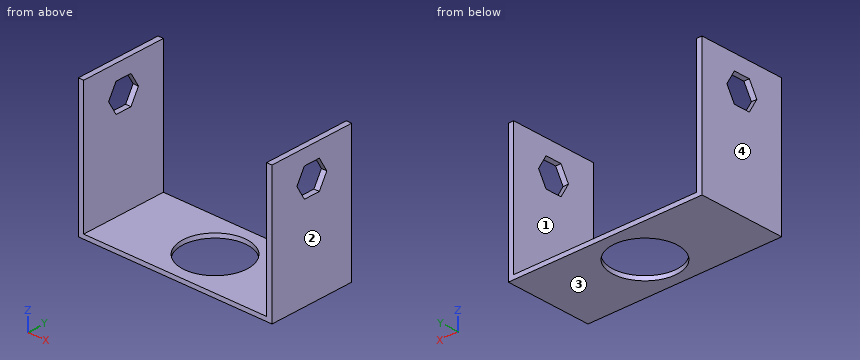
Autodesk Inventor part; units mm, degrees
ref_plane "Work Plane2" through (110.8745, -46.6041, 76.2) normal (1, 0, 0) x (0, 0, -1)
ref_plane "YZ Plane" through (0, 0, 0) normal (1, 0, 0) x (0, 1, 0)
ref_plane "XZ Plane" through (0, 0, 0) normal (0, 1, 0) x (-1, 0, 0)
sketch "Sketch1" plane through (0, 0, 0) normal (0, 0, 1) x (1, 0, 0)
  line L0 (-3.4255, 4.1959) -> (110.8745, 4.1959)
  line L1 (110.8745, 4.1959) -> (110.8745, -46.6041)
  line L2 (110.8745, -46.6041) -> (-3.4255, -46.6041)
  line L3 (-3.4255, -46.6041) -> (-3.4255, 4.1959)
  circle A0 centre (53.7245, -21.2041) radius 19.05
  line L4 (-0.2505, 4.1959) -> (-0.2505, -46.6041)
  line L5 (107.6995, -46.6041) -> (107.6995, 4.1959)
  point P0 (0, 0)
  dimension "d0" = 114.3
  dimension "d1" = 50.8
  dimension "d2" = 38.1
  dimension "d3" = 57.15
  dimension "d4" = 25.4
  dimension "d5" = 3.175
  dimension "d6" = 3.175
extrude "Extrusion1" add sketch "Sketch1" along normal blind 76.2 contours L0 L4 L2 L3 | L0 L1 L2 L5
extrude "Extrusion2" add sketch "Sketch1" against normal blind 2.54
ref_plane "Work Plane2" through (110.8745, -46.6041, 76.2) normal (1, 0, 0) x (0, 0, -1)
sketch "Sketch3" plane through (110.8745, -46.6041, 76.2) normal (1, 0, 0) x (0, 0, -1)
  line L0 (8.888, 20.6375) -> (8.888, 30.1625)
  line L1 (8.888, 30.1625) -> (17.1369, 34.925)
  line L2 (17.1369, 34.925) -> (25.3858, 30.1625)
  line L3 (25.3858, 30.1625) -> (25.3858, 20.6375)
  line L4 (25.3858, 20.6375) -> (17.1369, 15.875)
  line L5 (17.1369, 15.875) -> (8.888, 20.6375)
  line L6 (0, 0) -> (0, 50.8)
  line L7 (78.74, 0) -> (0, 0)
  point P0 (76.2, 46.6041)
  dimension "d12" = 9.525
  dimension "d13" = 9.525
  dimension "d14" = 120
  dimension "d15" = 9.525
  dimension "d16" = 120
  dimension "d17" = 9.525
  dimension "d18" = 120
  dimension "d19" = 8.888
  dimension "d20" = 15.875
extrude "Extrusion3" cut sketch "Sketch3" against normal blind 127
properties part number "shaft to bicep" material "CFRP"
Design review of the part built by this model. Coordinates are the model's own, in mm. Face numbers are marked on the shaded views. Round coordinates to 2 decimals unless told otherwise and drop trailing zeros. Loops run counter-clockwise (first coordinate to the right, second up) from the corner with the lowest first, then second, coordinate; pieces in that order, holes last. Notation, with made-up numbers: (59, 75) -> (82, 75) arc R15 cw to (82, 89) -> close; hole circle Ø1 at (59.25, -23). An arc over 180 degrees is marked (long way). Use one line per item in the form item = value. Start each with the question number.
Q1. We need section D-D on y = -9.5. Give the boundary of the cut face in (x, z).
Q2. We need section C-C on y = -15. Give the boundary of the cut face in (x, z), then the cut area to 3 significant figures.
Q3. Draft analysis for pull direction X (two halves, no side actions). For the marked faces 1, 2, 3 and 4, state which applies: +X half, -X half, draft (parallel to the pull), parting line (faces both ways), or undercut.
Q4. We need section B-B on x = 49.5. Give the boundary of the cut face in (y, z), then the cut area to 3 significant figures.
Q5. Wall thickness on line 1 along X through (y, z) = (-39, 3.5); line 2 along Z through (x, y) = (88, -10.5): over which ranges is each line inside the solid? List them lowest first. Write a range as [from, to].
Q6. We need section A-A on z = 4.5. Give the boundary of the cut face in (x, y), then the cut area to 3 significant figures.
Calculated:
q1.outline = (-3.43, -2.54) -> (38.69, -2.54) -> (38.69, 0) -> (-0.25, 0) -> (-0.25, 76.2) -> (-3.43, 76.2) -> close; (68.76, -2.54) -> (110.87, -2.54) -> (110.87, 76.2) -> (107.7, 76.2) -> (107.7, 0) -> (68.76, 0) -> close
q2.outline = (-3.43, -2.54) -> (35.71, -2.54) -> (35.71, 0) -> (-0.25, 0) -> (-0.25, 53.31) -> (-3.43, 53.31) -> close; (-3.43, 64.82) -> (-0.25, 64.82) -> (-0.25, 76.2) -> (-3.43, 76.2) -> close; (71.74, -2.54) -> (110.87, -2.54) -> (110.87, 53.31) -> (107.7, 53.31) -> (107.7, 0) -> (71.74, 0) -> close; (107.7, 64.82) -> (110.87, 64.82) -> (110.87, 76.2) -> (107.7, 76.2) -> close
q2.area = 610 mm²
q3.face_1 = undercut
q3.face_2 = +X half
q3.face_3 = draft
q3.face_4 = -X half
q4.outline = (-46.6, -2.54) -> (-39.78, -2.54) -> (-39.78, 0) -> (-46.6, 0) -> close; (-2.63, -2.54) -> (4.2, -2.54) -> (4.2, 0) -> (-2.63, 0) -> close
q4.area = 34.7 mm²
q5.line_1 = [-3.43, -0.25], [107.7, 110.87]
q5.line_2 = [-2.54, 0]
q6.outline = (-3.43, -46.6) -> (-0.25, -46.6) -> (-0.25, 4.2) -> (-3.43, 4.2) -> close; (107.7, -46.6) -> (110.87, -46.6) -> (110.87, 4.2) -> (107.7, 4.2) -> close
q6.area = 323 mm²
